from build123d import *

# Parameters (mm, degrees)
BOSS_EXTRUDE1_DEPTH            = 15
M5_CLEARANCE_HOLE1_D           = 5.5
M5_CLEARANCE_HOLE1_CSINK_D     = 5.55
M5_CLEARANCE_HOLE1_CSINK_ANGLE = 90
SKETCH8_W                      = 40
SKETCH8_H                      = 15
BOSS_EXTRUDE2_DEPTH            = 40
M5_CLEARANCE_HOLE2_D           = 5.5
M5_CLEARANCE_HOLE2_CSINK_D     = 5.55
M5_CLEARANCE_HOLE2_CSINK_ANGLE = 90
FILLET2_START                  = -32.15
FILLET2_DEPTH                  = 29.023091
FILLET2_START_2                = -1
FILLET2_2_DEPTH                = 16


with BuildPart() as part:
    # Sketch1 → Boss-Extrude1 (new body)
    with BuildSketch(Plane(origin=(0, 0, 0), x_dir=(1, 0, 0), z_dir=(0, 1, 0))):
        Polygon((0, 0), (40, 0), (40, 32.15), (60, 32.15), (60, 72.15), (-20, 72.15), (-20, 32.15), (0, 32.15), align=None)
    extrude(amount=BOSS_EXTRUDE1_DEPTH)

    # M5 Clearance Hole1 (through all)
    with Locations(Plane(origin=(0, 15, 0), x_dir=(1, 0, 0), z_dir=(0, 1, 0))):
        with Locations((-1.85, 52.15), (41.85, 52.15)):
            CounterSinkHole(M5_CLEARANCE_HOLE1_D / 2, M5_CLEARANCE_HOLE1_CSINK_D / 2, counter_sink_angle=M5_CLEARANCE_HOLE1_CSINK_ANGLE)

    # Sketch8 → Boss-Extrude2 (add)
    with BuildSketch(Plane(origin=(0, 15, 0), x_dir=(1, 0, 0), z_dir=(0, 1, 0))):
        with Locations((20, 22.5)):
            Rectangle(SKETCH8_W, SKETCH8_H)
    extrude(amount=BOSS_EXTRUDE2_DEPTH)

    # M5 Clearance Hole2 (through all)
    with Locations(Plane(origin=(0, 0, -30), x_dir=(-1, 0, 0), z_dir=(0, 0, -1))):
        with Locations((-10, 25), (-30, 45), (-30, 25), (-10, 45)):
            CounterSinkHole(M5_CLEARANCE_HOLE2_D / 2, M5_CLEARANCE_HOLE2_CSINK_D / 2, counter_sink_angle=M5_CLEARANCE_HOLE2_CSINK_ANGLE)

    # Fillet2: read off the stored shape, not the designer's step
    # Fillet2 outline → Fillet2 (cut)
    with BuildSketch(Plane.XY.offset(FILLET2_START)):
        with BuildLine():
            Line((40, 55), (30, 55))
            add(Edge.make_bspline(
                [(30, 55), (40, 55), (40, 45)],
                knots=[0, 0, 0, 1, 1, 1], degree=2, weights=[1, 0.707106781, 1]))
            Line((40, 45), (40, 55))
        make_face()
        with BuildLine():
            add(Edge.make_bspline(
                [(10, 55), (0, 55), (0, 45)],
                knots=[0, 0, 0, 1, 1, 1], degree=2, weights=[1, 0.707106781, 1]))
            Line((10, 55), (0, 55))
            Line((0, 55), (0, 45))
        make_face()
    extrude(amount=FILLET2_DEPTH, mode=Mode.SUBTRACT)

    # Fillet2 2 outline → Fillet2 2 (cut)
    with BuildSketch(Plane(origin=(0, 0, 0), x_dir=(1, 0, 0), z_dir=(0, 1, 0)).offset(FILLET2_START_2)):
        with BuildLine():
            Line((-20, 32.15), (-10, 32.15))
            add(Edge.make_bspline(
                [(-10, 32.15), (-20, 32.15), (-20, 42.15)],
                knots=[0, 0, 0, 1, 1, 1], degree=2, weights=[1, 0.707106781, 1]))
            Line((-20, 42.15), (-20, 32.15))
        make_face()
        with BuildLine():
            Line((-20, 72.15), (-20, 62.15))
            add(Edge.make_bspline(
                [(-20, 62.15), (-20, 72.15), (-10, 72.15)],
                knots=[0, 0, 0, 1, 1, 1], degree=2, weights=[1, 0.707106781, 1]))
            Line((-10, 72.15), (-20, 72.15))
        make_face()
        with BuildLine():
            Line((60, 72.15), (50, 72.15))
            add(Edge.make_bspline(
                [(50, 72.15), (60, 72.15), (60, 62.15)],
                knots=[0, 0, 0, 1, 1, 1], degree=2, weights=[1, 0.707106781, 1]))
            Line((60, 62.15), (60, 72.15))
        make_face()
        with BuildLine():
            add(Edge.make_bspline(
                [(10, 0), (0, 0), (0, 10)],
                knots=[0, 0, 0, 1, 1, 1], degree=2, weights=[1, 0.707106781, 1]))
            Line((0, 10), (0, 0))
            Line((0, 0), (10, 0))
        make_face()
        with BuildLine():
            Line((40, 0), (40, 10))
            add(Edge.make_bspline(
                [(40, 10), (40, 0), (30, 0)],
                knots=[0, 0, 0, 1, 1, 1], degree=2, weights=[1, 0.707106781, 1]))
            Line((30, 0), (40, 0))
        make_face()
        with BuildLine():
            add(Edge.make_bspline(
                [(60, 42.15), (60, 32.15), (50, 32.15)],
                knots=[0, 0, 0, 1, 1, 1], degree=2, weights=[1, 0.707106781, 1]))
            Line((50, 32.15), (60, 32.15))
            Line((60, 32.15), (60, 42.15))
        make_face()
    extrude(amount=FILLET2_2_DEPTH, mode=Mode.SUBTRACT)


solid = part.part
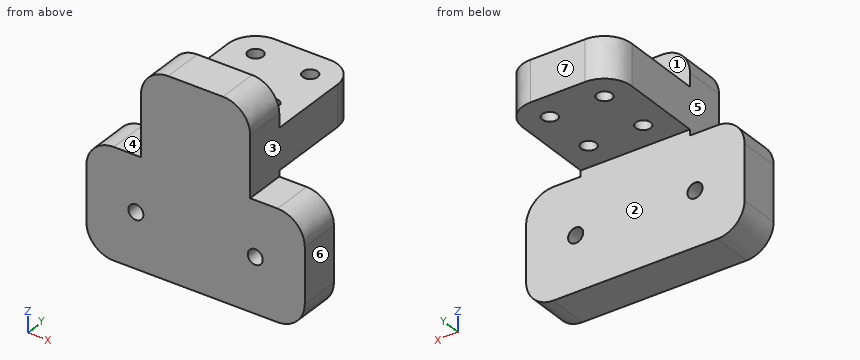
Design review of the part built by this model. Coordinates are the model's own, in mm. Face numbers are marked on the shaded views. A direction names the side the tool comes from. Round coordinates to 2 decimals unless told otherwise and drop trailing zeros. Loops run counter-clockwise (first coordinate to the right, second up) from the corner with the lowest first, then second, coordinate; pieces in that order, holes last. Notation, with made-up numbers: (40, 41.25) -> (97, 41.25) arc R16 ccw to (97, 55.25) -> close; hole circle Ø8 at (20, 35.5). An arc over 180 degrees is marked (long way). Use one line per item in the form item = value. Start each with the question number.
Q1. We need section A-A on z = -52.15. Give the boundary of the cut face in (x, y) (3 decimals), then the cut area to 4 significant figures.
Q2. Machinability: for the marked faces 1, 2, 3 and 4, which of the approach directions +Z, -Z, +X, -X, +Y, -Y give a long, thin tool a straight path to every point of the face, cutting with its end or side? Answer none if there is none.
Q3. Wall thickness on line 1 along Y through (x, z) = (30, -25.5); line 2 along X through (y, z) = (6.5, -52.15); line 3 along X through (y, z) = (25, -20): over which ranges is each line inside the solid? List them lowest first. Write a range as [from, to].
Q4. For pin 1 Ø1.5 at (x, z) = (40.5, -43) entering from +Y; pin 2 Ø6.5 at (x, y) = (10, 45) entering from +Z; pin 3 Ø10 at (x, y) = (-3.5, 23.5) entering from -Z, all flat-tipped, find the tip position at first contact; note any pin that passes through.
Q5. We need section C-C on y = 25. Give the boundary of the cut face in (x, z) (3 decimals).
Q6. Draft analysis for pull direction X (two halves, no side actions). For the marked faces 5, 6 and 7, state which applies: +X half, -X half, draft (parallel to the pull), parting line (faces both ways), or undercut.
Q7. We need section B-B on x = -1.85. Give the boundary of the cut face in (y, z) (3 decimals).
Q8. We need section D-D on x = 15.5. Give the boundary of the cut face in (y, z).
Calculated:
q1.outline = (-20, 0) -> (-4.6, 0) -> (-4.6, 14.975) -> (-4.625, 15) -> (-20, 15) -> close; (0.9, 0) -> (39.1, 0) -> (39.1, 14.975) -> (39.075, 15) -> (0.925, 15) -> (0.9, 14.975) -> close; (44.6, 0) -> (60, 0) -> (60, 15) -> (44.625, 15) -> (44.6, 14.975) -> close
q1.area = 1,035 mm²
q2.face_1 = +Z, +X, -X, +Y
q2.face_2 = -Z, +X, -X, +Y
q2.face_3 = +Z, +X, +Y, -Y
q2.face_4 = +Z, -X, +Y, -Y
q3.line_1 = [0, 22.25], [27.75, 42.25], [47.75, 55]
q3.line_2 = [-20, -4.6], [0.9, 39.1], [44.6, 60]
q3.line_3 = [0, 7.25], [12.75, 27.25], [32.75, 40]
q4.pin_1 = 15
q4.pin_2 = -15
q4.pin_3 = -30
q5.outline = (0, -30) -> (7.225, -30) -> (7.25, -29.975) -> (7.25, -15) -> (0, -15) -> close; (12.75, -29.975) -> (12.775, -30) -> (27.225, -30) -> (27.25, -29.975) -> (27.25, -15) -> (12.75, -15) -> close; (32.75, -29.975) -> (32.775, -30) -> (40, -30) -> (40, -15) -> (32.75, -15) -> close
q6.face_5 = -X half
q6.face_6 = +X half
q6.face_7 = draft
q7.outline = (0, -72.15) -> (15, -72.15) -> (15, -54.925) -> (14.975, -54.9) -> (0, -54.9) -> close; (0, -49.4) -> (14.975, -49.4) -> (15, -49.375) -> (15, -32.15) -> (0, -32.15) -> close
q8.outline = (0, -72.15) -> (15, -72.15) -> (15, -30) -> (55, -30) -> (55, -15) -> (15, -15) -> (15, 0) -> (0, 0) -> close
